The model under review builds one solid part; all positions refer to its coordinate system, in mm. Coordinates: 2 decimals unless noted, no trailing zeros. Write each loop counter-clockwise with the first axis right and the second up, starting at its lowest first coordinate (ties: lowest second). Pieces come first, ordered by that corner, then holes. Notation, with made-up numbers: (-27, 81.5) - (5, 81.5) arc R21 cw to (5, 96.5) - close; hole circle Ø9 at (-18, -19.75). An arc over 180 degrees is marked (long way). Return JSON: item names as keys, results as strings. Group by question number.
(1) We need section D-D on y = 6. State the section outline as (x, z) points (3 decimals), then the cut area to 3 significant figures.
(2) We need section A-A on y = -15. State the section outline as (x, z) points (3 decimals).
(3) To check wall thickness, follow L1, parallel to X at y = -12.5, z = 1.75 (3 decimals); L2, parallel to Y at x = 46, z = 0.35; L3, parallel to Y at x = -21.5, z = 1.9. State the ranges of each line that lie inside material, in increasing order. Write a range as from..to.
(4) We need section B-B on x = 52. State the section outline as (y, z) points, then the cut area to 3 significant figures.
(5) We need section C-C on x = -6.5. State the section outline as (y, z) points.
(6) For pin 1 Ø1.5 at (y, z) = (16, 2) entering from +X; pin 2 Ø2.5 at (x, y) = (-10.29, -10.46) entering from +Z; pin 3 Ø1.5 at (y, z) = (-18.5, 1.5) entering from +X (3 decimals), all flat-tipped, find the tip position at first contact; note any pin that passes through.
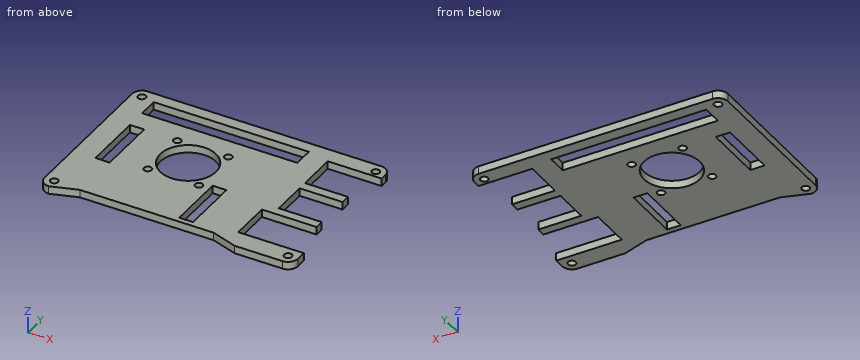
```python
from build123d import *

# Parameters (mm, degrees)
SKETCH1_R           = 1.524
SKETCH1_W           = 60.6932
SKETCH1_H           = 7.81
SKETCH1_W_2         = 5.588
SKETCH1_H_2         = 23.368
SKETCH1_W_3         = 5.4034
SKETCH1_H_3         = 22.6066
BOSS_EXTRUDE1_DEPTH = 3.048
SKETCH2_R           = 10.922
SKETCH2_R_2         = 1.4986
CUT_EXTRUDE1_DEPTH  = 72.310891511


with BuildPart() as part:
    # Sketch1 → Boss-Extrude1 (new body)
    with BuildSketch(Plane.XY):
        with BuildLine():
            Line((61.214907375, 24.068294304), (40.134807375, 24.068294304))
            Line((40.134807375, 24.068294304), (40.134807375, 8.658194304))
            Line((40.134807375, 8.658194304), (56.975007375, 8.658194304))
            Line((56.975007375, 8.658194304), (56.975007375, 4.997894304))
            Line((56.975007375, 4.997894304), (40.134807375, 4.997894304))
            Line((40.134807375, 4.997894304), (40.134807375, -9.121805696))
            Line((40.134807375, -9.121805696), (56.975007375, -9.121805696))
            Line((56.975007375, -9.121805696), (56.975007375, -12.628005696))
            Line((56.975007375, -12.628005696), (35.575007375, -12.628005696))
            Line((35.575007375, -12.628005696), (35.575007375, -28.627805696))
            Line((35.575007375, -28.627805696), (61.214907375, -28.627805696))
            Line((61.214907375, -28.627805696), (61.214907375, -32.613401529))
            ThreePointArc((61.214907375, -32.613401529), (60.108826144, -35.325305244), (57.405007375, -36.451005696))
            Line((57.405007375, -36.451005696), (38.714307375, -36.451005696))
            Line((38.714307375, -36.451005696), (28.474307375, -33.084405696))
            Line((28.474307375, -33.084405696), (-23.844892625, -33.084405696))
            Line((-23.844892625, -33.084405696), (-34.084892625, -36.451005696))
            ThreePointArc((-34.084892625, -36.451005696), (-36.778969461, -35.335082532), (-37.894892625, -32.641005696))
            Line((-37.894892625, -32.641005696), (-37.894892625, 26.697694304))
            ThreePointArc((-37.894892625, 26.697694304), (-36.778969461, 29.391771141), (-34.084892625, 30.507694304))
            Line((-34.084892625, 30.507694304), (57.404932375, 30.507694304))
            ThreePointArc((57.404932375, 30.507694304), (60.103884597, 29.386886916), (61.214907375, 26.683892153))
            Line((61.214907375, 26.683892153), (61.214907375, 24.068294304))
        make_face()
        with Locations(Location((57.405007375, -32.641005696, 0), (0, 0, 180))):
            Circle(SKETCH1_R, mode=Mode.SUBTRACT)
        with Locations(Location((-34.084892625, -32.641005696, 0), (0, 0, 180))):
            Circle(SKETCH1_R, mode=Mode.SUBTRACT)
        with Locations(Location((-34.084892625, 26.697694304, 0), (0, 0, 180))):
            Circle(SKETCH1_R, mode=Mode.SUBTRACT)
        with Locations(Location((57.404932375, 26.697694304, 0), (0, 0, 180))):
            Circle(SKETCH1_R, mode=Mode.SUBTRACT)
        with Locations((1.341707375, 21.991994304)):
            Rectangle(SKETCH1_W, SKETCH1_H, mode=Mode.SUBTRACT)
        with Locations((-26.210892625, -1.882805696)):
            Rectangle(SKETCH1_W_2, SKETCH1_H_2, mode=Mode.SUBTRACT)
        with Locations((16.546707375, -19.663505696)):
            Rectangle(SKETCH1_W_3, SKETCH1_H_3, mode=Mode.SUBTRACT)
    extrude(amount=BOSS_EXTRUDE1_DEPTH)

    # Sketch2 → Cut-Extrude1 (cut, through all)
    with BuildSketch(Plane.XY.offset(3.048)):
        with Locations((-0.302892625, -0.480305696)):
            Circle(SKETCH2_R)
        with Locations((-10.285092625, -10.462505696)):
            Circle(SKETCH2_R_2)
        with Locations((-10.285092625, 9.501894304)):
            Circle(SKETCH2_R_2)
        with Locations((9.679307375, -10.462505696)):
            Circle(SKETCH2_R_2)
        with Locations((9.679307375, 9.501894304)):
            Circle(SKETCH2_R_2)
    extrude(amount=-CUT_EXTRUDE1_DEPTH, mode=Mode.SUBTRACT)


solid = part.part
```
Ans:
{
 "1": {"outline": "(-37.895, 0) - (-29.005, 0) - (-29.005, 3.048) - (-37.895, 3.048) - close; (-23.417, 0) - (-9.095, 0) - (-9.095, 3.048) - (-23.417, 3.048) - close; (8.489, 0) - (56.975, 0) - (56.975, 3.048) - (8.489, 3.048) - close", "area": "219 mm²"},
 "2": {"outline": "(-37.895, 0) - (13.845, 0) - (13.845, 3.048) - (-37.895, 3.048) - close; (19.248, 0) - (35.575, 0) - (35.575, 3.048) - (19.248, 3.048) - close"},
 "3": {"L1": "-37.895..-29.005, -23.417..13.845, 19.248..56.975", "L2": "-36.45..-28.63, -12.63..-9.12, 5..8.66, 24.07..30.51", "L3": "-33.08..18.09, 25.9..30.51"},
 "4": {"outline": "(-36.45, 0) - (-28.63, 0) - (-28.63, 3.05) - (-36.45, 3.05) - close; (-12.63, 0) - (-9.12, 0) - (-9.12, 3.05) - (-12.63, 3.05) - close; (5, 0) - (8.66, 0) - (8.66, 3.05) - (5, 3.05) - close; (24.07, 0) - (30.51, 0) - (30.51, 3.05) - (24.07, 3.05) - close", "area": "65.3 mm²"},
 "5": {"outline": "(-33.08, 0) - (-9.47, 0) - (-9.47, 3.05) - (-33.08, 3.05) - close; (8.51, 0) - (18.09, 0) - (18.09, 3.05) - (8.51, 3.05) - close; (25.9, 0) - (30.51, 0) - (30.51, 3.05) - (25.9, 3.05) - close"},
 "6": {"pin 1": "x = 40.13", "pin 2": "through", "pin 3": "x = 35.575"}
}
